For this review, take the finished solid that the model builds, in its own axes (mm). A direction names the side the tool comes from. Give positions to 0.01 mm unless a question says otherwise; leave off trailing zeros. Write each loop counter-clockwise with the first axis right and the second up, starting at its lowest first coordinate (ties: lowest second). Pieces come first, ordered by that corner, then holes.
from build123d import *

# Parameters (mm, degrees)
SKETCH1_R           = 72.5
BOSS_EXTRUDE1_DEPTH = 25
SKETCH2_R           = 17.5
CUT_EXTRUDE1_DEPTH  = 106.534354596
SKETCH3_R           = 6.721755304
CUT_EXTRUDE2_DEPTH  = 24.234624
CIRPATTERN1_START   = 0.765375699
CIRPATTERN1_DEPTH   = 24.234624301


# Read off the part's stored shape, not the designer's step: CirPattern1
with BuildPart() as part:
    # Sketch1 → Boss-Extrude1 (new body)
    with BuildSketch(Plane(origin=(0, 0, 0), x_dir=(1, 0, 0), z_dir=(0, 1, 0))):
        with Locations(Location((0, 0, 0), (0, 0, 270))):
            Circle(SKETCH1_R)
    extrude(amount=BOSS_EXTRUDE1_DEPTH)

    # Sketch2 → Cut-Extrude1 (cut, through all)
    with BuildSketch(Plane(origin=(0, 0, 0), x_dir=(1, 0, 0), z_dir=(0, 1, 0))):
        with Locations(Location((0, 0, 0), (0, 0, 270))):
            Circle(SKETCH2_R)
    extrude(amount=CUT_EXTRUDE1_DEPTH, mode=Mode.SUBTRACT)

    # Sketch3 → Cut-Extrude2 (cut)
    with BuildSketch(Plane(origin=(0, 25, 0), x_dir=(1, 0, 0), z_dir=(0, 1, 0))):
        with Locations((-17.104622237, 0)):
            Circle(SKETCH3_R)
    extrude(amount=-CUT_EXTRUDE2_DEPTH, mode=Mode.SUBTRACT)

    # CirPattern1 outline → CirPattern1 (cut)
    with BuildSketch(Plane(origin=(0, 0, 0), x_dir=(1, 0, 0), z_dir=(0, 1, 0)).offset(CIRPATTERN1_START)):
        with BuildLine():
            ThreePointArc((2.325576061, 17.344788727), (8.75, 15.155444566), (13.85823963, 10.686402311))
            ThreePointArc((13.85823963, 10.686402311), (11.91318877, 20.63424823), (2.325576061, 17.344788727))
        make_face()
        with BuildLine():
            ThreePointArc((13.85823963, -10.686402311), (8.75, -15.155444566), (2.325576061, -17.344788727))
            ThreePointArc((2.325576061, -17.344788727), (11.91318877, -20.63424823), (13.85823963, -10.686402311))
        make_face()
    extrude(amount=CIRPATTERN1_DEPTH, mode=Mode.SUBTRACT)


solid = part.part
(1) Tool access review of faces 1 (the flat face through (10, 0.765, 17)), 2 (the cylindrical face through (-10.648, 12.325, -13.887)): name each direction out of +Z, -Z, +X, -X, +Y, -Y from which nothing blocks a thin tool from reaching the whole face with its end or side.
(2) The part is to be moulded in two halves that separate along Z. For faces 3 (the flat face through (-15, 25, 15)), 4 (the cylindrical face through (-23.824, 13.052, -0.161)), 5 (the cylindrical face through (21.78, 12.32, 69.15)), say which applies: +Z half, -Z half, draft (parallel to the pull), parting line (faces both ways), or undercut.
(3) We need section D-D (z = -50). Write out the cut boundary in (x, y).
(4) We need section A-A (z = 0). Write out the cut boundary in (x, y).
(5) For L1, parallel to X at y = 18, z = 0; L2, parallel to Z at x = 14, y = 7.5; L3, parallel to X at y = 14, z = 7, list the stretches that pass through material, from the lowest coordinate up.
(6) We need section B-B (x = 0). Write out the cut boundary in (y, z).
(7) Clearance check with flat-ended pins moving along their axes: pin 1 Ø6 at (y, z) = (21, 34) entering from -X; pin 2 Ø4 at (y, z) = (17, 41) entering from +X; pin 3 Ø2.5 at (x, z) = (-19, 3) entering from +Y. State where each tip first meets the part, or that it passes through.
(8) We need section C-C (y = 12.25). Write out the cut boundary in (x, z), and give its area (3 significant figures).
The answers:
1. face 1: +Y
1. face 2: +Y, -Y
2. face 3: draft
2. face 4: undercut
2. face 5: parting line
3. outline: (-52.5, 0) - (52.5, 0) - (52.5, 25) - (-52.5, 25) - close
4. outline: (-72.5, 0) - (-17.5, 0) - (-17.5, 0.77) - (-23.83, 0.77) - (-23.83, 25) - (-72.5, 25) - close; (17.5, 0) - (72.5, 0) - (72.5, 25) - (17.5, 25) - close
5. L1: x = -72.5 to -23.83, 17.5 to 72.5
5. L2: z = -71.14 to -18.75, -10.88 to -10.5, 10.5 to 10.88, 18.75 to 71.14
5. L3: x = -72.16 to -16.04, 16.04 to 72.16
6. outline: (0, -72.5) - (25, -72.5) - (25, -17.5) - (0, -17.5) - close; (0, 17.5) - (25, 17.5) - (25, 72.5) - (0, 72.5) - close
7. pin 1: stops at x = -65.54
7. pin 2: stops at x = 61.12
7. pin 3: stops at y = 0.77
8. outline: circle Ø145 at (0, 0); hole (-16.18, -6.66) arc R17.5 ccw to (2.33, -17.34) arc R6.72 ccw (long way) to (13.86, -10.69) arc R17.5 ccw to (13.86, 10.69) arc R6.72 ccw (long way) to (2.33, 17.34) arc R17.5 ccw to (-16.18, 6.66) arc R6.72 ccw (long way) to start
8. area: 15,300 mm2
